Autodesk Inventor part; units mm, degrees
ref_plane "YZ Plane" through (0, 0, 0) normal (1, 0, 0) x (0, 1, 0)
ref_plane "XZ Plane" through (0, 0, 0) normal (0, 1, 0) x (-1, 0, 0)
ref_plane "XY Plane" through (0, 0, 0) normal (0, 0, 1) x (1, 0, 0)
sketch "Sketch1" plane through (0, 0, 0) normal (0, 1, 0) x (-1, 0, 0)
  line L0 (10, 10) -> (-10, 10)
  line L1 (-10, 10) -> (-10, -10)
  line L2 (-10, -10) -> (10, -10)
  line L3 (10, -10) -> (10, 10)
  line L4 (10, 10) -> (-10, -10) construction
  line L5 (-10, 10) -> (10, -10) construction
  point P0 (0, 0)
  dimension "d0" = 20
  dimension "d1" = 20
extrude "Extrusion1" add sketch "Sketch1" along normal blind 20
sketch "Sketch2" plane through (0, 20, 0) normal (0, 1, 0) x (1, 0, 0)
  circle A0 centre (0, 0) radius 15
  dimension "d4" = 30
extrude "Extrusion2" add sketch "Sketch2" along normal blind 30
sketch "Sketch3" plane through (0, 50, 0) normal (0, 1, 0) x (1, 0, 0)
  line L0 (-15, -50) -> (15, -50)
  line L1 (15, -50) -> (15, 50)
  line L2 (15, 50) -> (-15, 50)
  line L3 (-15, 50) -> (-15, -50)
  line L4 (-15, -50) -> (15, 50) construction
  line L5 (15, -50) -> (-15, 50) construction
  point P0 (0, 0)
  dimension "d7" = 30
  dimension "d8" = 100
extrude "Extrusion3" add sketch "Sketch3" along normal blind 5
sketch "Sketch4" plane through (0, 55, 0) normal (0, 1, 0) x (1, 0, 0)
  arc A0 (-3, 41.5) -> (-3, 28.5) centre (-3, 35) ccw
  arc A1 (3, 28.5) -> (3, 41.5) centre (3, 35) ccw
  line L0 (-3, 28.5) -> (3, 28.5)
  line L1 (-3, 41.5) -> (3, 41.5)
  point P0 (0, 0)
  dimension "d11" = 13
  dimension "d12" = 13
  dimension "d13" = 3
  dimension "d14" = 3
  dimension "d15" = 35
extrude "Extrusion4" cut sketch "Sketch4" against normal blind 5
fillet "Fillet1" radius 10 2 edges at (-15, 52.5, -50) (15, 52.5, -50)
sketch "Sketch5" plane through (0, 55, 0) normal (0, 1, 0) x (1, 0, 0)
  circle A0 centre (0, -39.6695) radius 1
  point P0 (0, 0)
  dimension "d19" = 2
extrude "Extrusion5" cut sketch "Sketch5" against normal blind 5
sketch "Sketch6" plane through (0, 0, 0) normal (0, -1, 0) x (1, 0, 0)
  circle A0 centre (-14.1421, 14.1421) radius 2.5
  circle A1 centre (-14.1421, -14.1421) radius 2.5
  line L0 (0, 0) -> (-14.1421, 14.1421)
  line L1 (0, 0) -> (0, -20)
  line L2 (0, 0) -> (-14.1421, -14.1421)
  circle A2 centre (0, -20) radius 2.5
  circle A3 centre (0, 0) radius 25
  line L3 (0, 0) -> (14.1421, 14.1421)
  circle A4 centre (14.1421, 14.1421) radius 2.5
  line L4 (0, 0) -> (14.1421, -14.1421)
  circle A5 centre (14.1421, -14.1421) radius 2.5
  line L5 (-10, 10) -> (10, 10)
  line L6 (10, 10) -> (10, -10)
  line L7 (10, -10) -> (-10, -10)
  line L8 (-10, -10) -> (-10, 10)
  line L9 (-10, 10) -> (10, -10) construction
  line L10 (10, 10) -> (-10, -10) construction
  dimension "d22" = 20
  dimension "d23" = 20
  dimension "d24" = 135
  dimension "d25" = 5
  dimension "d26" = 5
  dimension "d27" = 20
  dimension "d28" = 90
  dimension "d29" = 5
  dimension "d30" = 20
  dimension "d31" = 90
  dimension "d32" = 5
  dimension "d33" = 20
  dimension "d34" = 90
  dimension "d35" = 5
  dimension "d36" = 20
  dimension "d37" = 20
extrude "Extrusion6" add sketch "Sketch6" against normal blind 10
sketch "Sketch7" plane through (0, 55, 0) normal (0, 1, 0) x (1, 0, 0)
  arc A0 (-3, 41.5) -> (-3, 28.5) centre (-3, 35) ccw
  arc A1 (3, 28.5) -> (3, 41.5) centre (3, 35) ccw
  line L0 (-3, 28.5) -> (3, 28.5)
  line L1 (-3, 41.5) -> (3, 41.5)
  point P0 (0, 0)
  dimension "d40" = 13
  dimension "d41" = 13
extrude "Extrusion7" add sketch "Sketch7" along normal blind 15 and the other way blind 5
sketch "Sketch8" plane through (0, 70, 0) normal (0, 1, 0) x (1, 0, 0)
  line L0 (-2.5, 25) -> (2.5, 25)
  line L1 (2.5, 25) -> (2.5, 45)
  line L2 (2.5, 45) -> (-2.5, 45)
  line L3 (-2.5, 45) -> (-2.5, 25)
  line L4 (-2.5, 25) -> (2.5, 45) construction
  line L5 (2.5, 25) -> (-2.5, 45) construction
  arc A0 (-2.8422, 41.5) -> (-2.8422, 28.5) centre (-2.8422, 35) ccw construction
  arc A1 (3.1578, 28.5) -> (3.1578, 41.5) centre (3.1578, 35) ccw construction
  line L6 (-2.8422, 28.5) -> (3.1578, 28.5) construction
  line L7 (-2.8422, 41.5) -> (3.1578, 41.5) construction
  point P0 (0, 0)
  point P1 (0, 35)
  point P2 (0, 35)
  point P3 (0, 35)
  dimension "d46" = 5
  dimension "d47" = 20
  dimension "d48" = 13
  dimension "d49" = 13
  dimension "d50" = 35
  dimension "d51" = 0
  dimension "d52" = 0
extrude "Extrusion8" add sketch "Sketch8" along normal blind 30
sketch "Sketch9" plane through (2.5, 70, -25) normal (1, 0, 0) x (0, 0, -1)
  line L0 (0, 0) -> (0, 30) construction
  line L1 (16.5, 0) -> (20, 0)
  line L2 (0, 30) -> (20, 30) construction
  line L3 (20, 30) -> (20, 0) construction
  line L4 (20, 0) -> (0, 0) construction
  line L5 (0, 0) -> (0, 30) construction
  arc A0 (16.5, 19) -> (3.5, 19) centre (10, 19) ccw
  arc A1 (3.5, 13) -> (16.5, 13) centre (10, 13) ccw
  line L6 (3.5, 13) -> (3.5, 19)
  line L7 (16.5, 19) -> (16.5, 13)
  point P0 (-25, -70)
  point P1 (18.25, 0)
  dimension "d55" = 13
  dimension "d56" = 13
  dimension "d57" = 6
  dimension "d58" = 13
extrude "Extrusion9" cut sketch "Sketch9" against normal blind 30
fillet "Fillet2" radius 10 2 edges at (0, 100, -45) (0, 100, -25)
sketch "Sketch10" plane through (0, 50, 0) normal (0, -1, 0) x (1, 0, 0)
  circle A0 centre (0, 39.6695) radius 1
  line L0 (0, 0) -> (0, 39.6695) construction
  circle A1 centre (0, 39.6695) radius 1
extrude "Extrusion10" add sketch "Sketch10" against normal blind 23
sketch "Sketch11" plane through (2.5, 70, -25) normal (1, 0, 0) x (0, 0, -1)
  arc A0 (16.5, 19) -> (3.5, 19) centre (10, 19) ccw
  arc A1 (3.5, 13) -> (16.5, 13) centre (10, 13) ccw
  line L0 (3.5, 13) -> (3.5, 19)
  line L1 (16.5, 19) -> (16.5, 13)
  point P0 (-25, -70)
  dimension "d65" = 13
  dimension "d66" = 13
  dimension "d67" = 6
extrude "Extrusion11" add sketch "Sketch11" along normal blind 15 and the other way blind 5
sketch "Sketch13" plane through (17.5, 70, -25) normal (1, 0, 0) x (0, 0, -1)
  line L0 (3.5, 13) -> (3.5, 19) construction
  arc A0 (3.5, 13) -> (16.5, 13) centre (10, 13) ccw
  line L1 (3.5, 19) -> (16.5, 19) construction
  line L2 (16.5, 19) -> (16.5, 13) construction
  line L3 (16.5, 13) -> (3.5, 13) construction
  line L4 (3.5, 13) -> (3.5, 19) construction
  circle A1 centre (10, 16) radius 22.5
  point P0 (-25, -70)
  dimension "d76" = 45
extrude "Extrusion13" add sketch "Sketch13" along normal blind 5
properties part number "herramienta5"
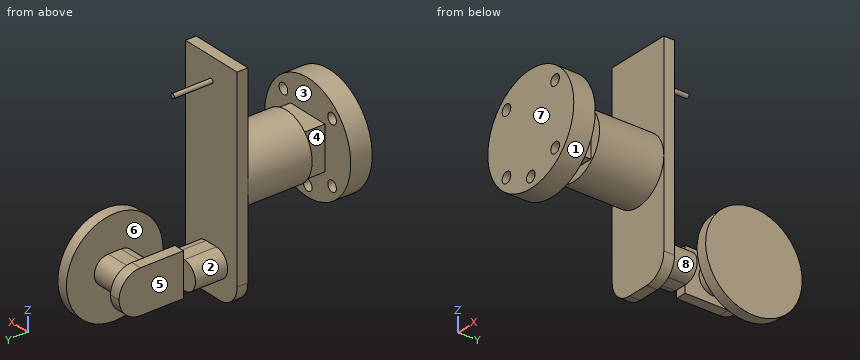
Geometry check sheet. Reference: the model listing, model coordinates, mm. Face numbers are marked on the shaded views. A direction names the side the tool comes from. Coordinates: 2 decimals unless noted, no trailing zeros. Write each loop counter-clockwise with the first axis right and the second up, starting at its lowest first coordinate (ties: lowest second). Pieces come first, ordered by that corner, then holes. Notation, with made-up numbers: M -16.5,31.25 L -3.5,31.25 A19 cw -3.5,61.25 Z; hole C 61,13.5 d6. An arc over 180 degrees is marked long. Answer as a JSON object with one key per item and string values.
1. Scan lines: L1, parallel to Y at x = -12, z = 2; L2, parallel to Z at x = 0, y = 5; L3, parallel to Y at x = 6.5, z = -4. Record each from-to range of solid material in increasing order.
Answers below:
{"L1": "y = 0 to 10, 20 to 55", "L2": "z = -25 to -22.5, -17.5 to 25", "L3": "y = 0 to 55"}
2. Section check A-A, the plane y = 24. Enter the section's corners in (x, z).
Answers below:
{"outline": "C 0,0 d30"}
3. Draft check along Y on the marked faces 6, 7 and 8. Enter one of: released by +Y, released by -Y, zero draft, split by the parting line, or undercut.
Answers below:
{"face 6": "zero draft", "face 7": "released by -Y", "face 8": "undercut"}
4. Go/stop test with flat-tipped pins: pin 1 Ø22 at (y, z) = (86, -39.5) entering from +X; pin 2 Ø4 at (y, z) = (52, -10) entering from -X; pin 3 Ø11 at (x, y) = (-5, 16.5) entering from -Z. Record where each tip stops, or that it passes through.
Answers below:
{"pin 1": "stops at x = 22.5", "pin 2": "stops at x = -15", "pin 3": "stops at z = -14.98"}
5. Tool access check on the marked faces 1, 2, 3, 4 and 5. Record the directions out of +Z, -Z, +X, -X, +Y, -Y that give a thin tool (end or side, any length) a straight path to the whole face; none if there is none.
Answers below:
{"face 1": "-Y", "face 2": "-X, +Y", "face 3": "none", "face 4": "+Z, -Z, -X", "face 5": "+Z, -Z, -X, +Y"}
